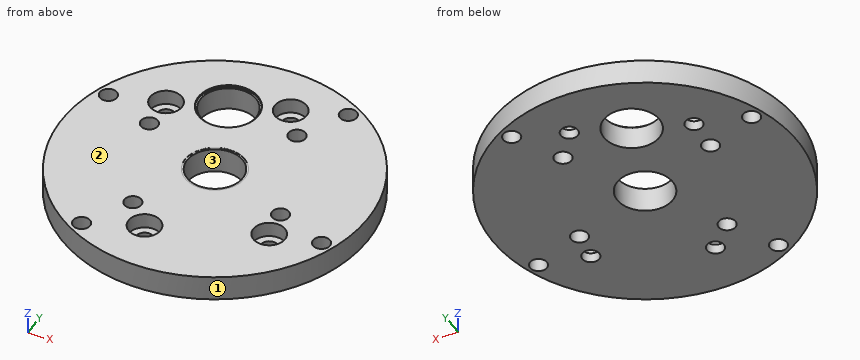
Autodesk Inventor part; units mm, degrees
ref_plane "Work Plane1" through (-28.6125, -68.0536, -6.35) normal (0, 0, -1) x (0, 1, 0)
ref_plane "YZ Plane" through (0, 0, 0) normal (1, 0, 0) x (0, 1, 0)
ref_plane "XZ Plane" through (0, 0, 0) normal (0, 1, 0) x (-1, 0, 0)
ref_plane "Work Plane1" through (-28.6125, -68.0536, -6.35) normal (0, 0, -1) x (0, 1, 0)
sketch "Sketch1" plane through (0, 0, 0) normal (0, 0, 1) x (1, 0, 0)
  circle A0 centre (39.4411, 0) radius 38.42
  circle A1 centre (28.7179, -18.967) radius 2.975 construction
  circle A2 centre (18.97, 7.4611) radius 2.975 construction
  circle A3 centre (59.9122, -7.4611) radius 2.975 construction
  circle A4 centre (50.1643, 18.967) radius 2.875 construction
  circle A5 centre (39.4411, 0) radius 7
  circle A6 centre (31.7519, 21.0389) radius 7
  circle A7 centre (59.9122, -7.4611) radius 2.15
  circle A8 centre (50.1643, 18.967) radius 2.15
  circle A9 centre (18.97, 7.4611) radius 2.15
  circle A10 centre (28.7179, -18.967) radius 2.15
  point P0 (0, 0)
extrude "Extrusion1" add sketch "Sketch1" against normal up to surface (6.35 mm away)
ref_plane "Work Plane2" through (39.4411, 0, -4.95) normal (0, 0, -1) x (-0.4776, -0.8786, 0)
sketch "Sketch3" plane through (39.4411, 0, 0) normal (0, 0, 1) x (1, 0, 0)
  circle A0 centre (0, 0) radius 7.5
  circle A1 centre (-7.6892, 21.0389) radius 7 construction
  circle A2 centre (-7.6892, 21.0389) radius 7.5
  point P0 (-39.4411, 0)
  dimension "d10" = 15
extrude "Extrusion3" cut sketch "Sketch3" against normal blind 0.5 contours A2
sketch "Sketch5" plane through (39.4411, 0, 0) normal (0, 0, 1) x (1, 0, 0)
  circle A0 centre (0, 0) radius 7.3 construction
  circle A1 centre (0, 0) radius 7.5
  point P0 (-39.4411, 0)
  dimension "d11" = 15
extrude "Extrusion4" cut sketch "Sketch5" against normal blind 0.05
sketch "Sketch6" plane through (39.4411, 0, 0) normal (0, 0, 1) x (1, 0, 0)
  circle A0 centre (20.4711, -7.4611) radius 2.975 construction
  circle A1 centre (10.7232, 18.967) radius 2.975 construction
  circle A2 centre (-20.4711, 7.4611) radius 2.975 construction
  circle A3 centre (-10.7232, -18.967) radius 2.975 construction
  line L0 (20.4711, -7.4611) -> (-20.4711, 7.4611) construction
  line L1 (-10.7232, -18.967) -> (10.7232, 18.967) construction
  circle A4 centre (17.4307, 30.8313) radius 2.15
  circle A5 centre (-17.4307, -30.8313) radius 2.15
  line L2 (17.4307, 30.8313) -> (-17.4307, -30.8313) construction
  circle A6 centre (0, 0) radius 38.42 construction
  circle A7 centre (33.2762, -12.1282) radius 2.15
  circle A8 centre (-33.2762, 12.1282) radius 2.15
  line L3 (33.2762, -12.1282) -> (-33.2762, 12.1282) construction
  point P0 (-39.4411, 0)
  dimension "d16" = 4.3
  dimension "d17" = 4.3
  dimension "d18" = 35.4175
  dimension "d19" = 35.4175
  dimension "d20" = 0
  dimension "d21" = 4.3
  dimension "d22" = 4.3
  dimension "d23" = 0
  dimension "d24" = 35.4175
  dimension "d25" = 35.4175
  dimension "d26" = 0
extrude "Extrusion5" cut sketch "Sketch6" against normal up to surface (6.35 mm away)
sketch "Sketch7" plane through (39.4411, 0, 0) normal (0, 0, 1) x (1, 0, 0)
  circle A0 centre (5.337, 26.1691) radius 2.15 construction
  circle A1 centre (-20.7154, 15.9087) radius 2.15 construction
  circle A2 centre (5.337, 26.1691) radius 4
  circle A3 centre (-20.7154, 15.9087) radius 4
  circle A4 centre (-4.5849, -25.0485) radius 2.15 construction
  circle A5 centre (21.4675, -14.7881) radius 2.15 construction
  circle A6 centre (21.4675, -14.7881) radius 4
  circle A7 centre (-4.5849, -25.0485) radius 4
  point P0 (-39.4411, 0)
  dimension "d29" = 8
  dimension "d30" = 8
  dimension "d37" = 8
  dimension "d38" = 8
  dimension "d39" = 0
  dimension "d40" = 0
extrude "Extrusion6" cut sketch "Sketch7" against normal blind 3.81
sketch "Sketch8" plane through (44.7781, 26.1691, -3.81) normal (0, 0, 1) x (1, 0, 0)
  circle A0 centre (0, 0) radius 4 construction
  circle A1 centre (-26.0523, -10.2604) radius 4 construction
  circle A2 centre (0, 0) radius 2.15
  circle A3 centre (-26.0523, -10.2604) radius 2.15
  circle A4 centre (-9.9218, -51.2176) radius 2.15
  circle A5 centre (16.1305, -40.9573) radius 2.15
  point P0 (-44.7781, -26.1691)
  dimension "d33" = 4.3
  dimension "d34" = 4.3
extrude "Extrusion7" cut sketch "Sketch8" against normal through all
equation "\"d19\" = d18"
equation "\"d24\" = d18"
equation "\"d25\" = d18"
properties part number "Inner_Pod_Holder"
Build history of the part. All positions in model axes, mm. Face numbers are marked on the shaded views. Round coordinates to 2 decimals unless told otherwise and drop trailing zeros. Write each loop counter-clockwise with the first axis right and the second up, starting at its lowest first coordinate (ties: lowest second). Pieces come first, ordered by that corner, then holes. Notation, with made-up numbers: (22.25, -22) - (62.25, -22) arc R7 cw to (62.25, -14) - close; hole circle Ø1 at (75, 5.5). An arc over 180 degrees is marked (long way). Write each question's results on one line, items separated by ' | '. Start each with the question number.
Item 1: Saw through at A-A (y = 0). Write the cut outline in (x, z).
Item 2: Drop flat-ended pins along their axis: P1, Ø1.5, axis at y = -10, z = -1.5, coming from the +X side; P2, Ø16.5, axis at x = 31, y = 18.5, coming from the +Z side; P3, Ø2, axis at x = 35.5, z = -1.5, coming from the -Y side; P4, Ø2.5, axis at x = 62.5, y = -13, coming from the +Z side. Give the stop position or say it passes through.
Item 3: Wall check: L1, parallel to X at y = 29.5, z = -3.75; L2, parallel to X at y = -6, z = -3; L3, parallel to Y at x = 18.97, z = -2.5. Give the ranges that are in metal, low to high. Write a range as [from, to].
Item 4: Mould opens along Y. For the marked faces 1, 2 and 3 say: pulls with the +Y half, pulls with the -Y half, needs draft (parallel to the pull), parting line crosses it, or undercut.
Item 5: Saw through at C-C (z = -2.5). State how many separate pieces and enclosed holes the cut face has, and give its area (3 significant figures).
Item 6: Saw through at B-B (x = 18.97). Write the cut outline in (y, z), and give its area (3 significant figures).
Results are:
1) outline: (1.02, -6.35) - (32.44, -6.35) - (32.44, -0.05) - (31.94, -0.05) - (31.94, 0) - (1.02, 0) - close; (46.44, -6.35) - (77.86, -6.35) - (77.86, 0) - (46.94, 0) - (46.94, -0.05) - (46.44, -0.05) - close
2) P1: stops at x = 76.73 | P2: stops at z = 0 | P3: stops at y = -38.31 | P4: stops at z = -3.81
3) L1: x = [14.83, 42.56], [46.99, 55.18], [58.56, 64.06] | L2: x = [1.49, 35.84], [43.05, 58.33], [61.49, 77.39] | L3: y = [-32.51, 5.31], [9.61, 11.92], [19.9, 32.51]
4) face 1: parting line crosses it | face 2: needs draft | face 3: undercut
5) separate pieces: 1 | enclosed holes: 14 | area: 4,010 mm²
6) outline: (-32.51, -6.35) - (5.31, -6.35) - (5.31, 0) - (-32.51, 0) - close; (9.61, -6.35) - (13.77, -6.35) - (13.77, -3.81) - (11.92, -3.81) - (11.92, 0) - (9.61, 0) - close; (18.04, -6.35) - (32.51, -6.35) - (32.51, 0) - (19.9, 0) - (19.9, -3.81) - (18.04, -3.81) - close | area: 344 mm²
